CAD build for the part. Positions are in the model's coordinates, mm. A direction names the side the tool comes from. Give positions to 0.01 mm unless a question says otherwise; leave off trailing zeros. Loops run counter-clockwise (first coordinate to the right, second up) from the corner with the lowest first, then second, coordinate; pieces in that order, holes last.
Solid Edge part; units mm, degrees
sketch "Sketch1" plane through (0, 0, 0) normal (0, 0, 1) x (1, 0, 0)
  line L0 (-1.8475, 3.2) -> (1.8475, 3.2)
  line L1 (1.8475, 3.2) -> (3.695, 0)
  line L2 (3.695, 0) -> (1.8475, -3.2)
  line L3 (1.8475, -3.2) -> (-1.8475, -3.2)
  line L4 (-1.8475, -3.2) -> (-3.695, 0)
  line L5 (-3.695, 0) -> (-1.8475, 3.2)
extrude "Protrusion1" add sketch "Sketch1" along normal blind 0.5
sketch "Sketch2" plane through (0, 0, 0.5) normal (0, 0, 1) x (1, 0, 0)
  circle A0 centre (0, 0) radius 2.7
extrude "Ausprägung_2" add sketch "Sketch2" along normal blind 5.5
hole "Bohrung_1" at (0, 0, 6) direction (0, 0, -1) diameter 3 depth 5
chamfer "Fase_1" distance 0.5 angle 45 1 edges at (0, 1.5, 6)
1. Tool access for faces 5 (the face through (-0.585, 2.636, 3.212)), 6 (the face through (0, 0, 0)): list every direction of +Z, -Z, +X, -X, +Y, -Y with a clear straight run to the whole face (end or side of a thin tool).
Responses:
face 5: +Z
face 6: -Z, +X, -X, +Y, -Y
2. Drop flat-ended pins along their axis: pin 1 (2 mm diameter, centred on y = -0.5, z = 3.5, fed in from -X); pin 2 (2.5 mm diameter, centred on x = -0.5, y = 0.5, fed in from +Z). Give the stop position or say it passes through.
Responses:
pin 1: stops at x = -2.7
pin 2: stops at z = 5.96
3. Pull direction X, two halves, no side cores. Call faces 1 (the face through (-3, 0, 0.5)), 2 (the face through (2.784, -1.578, 0.246)), 3 (the face through (-0.07, 1.5, 3.22)), 4 (the face through (-2.784, 1.578, 0.246)): released by +X, released by -X, zero draft, split by the parting line, or undercut.
Responses:
face 1: zero draft
face 2: released by +X
face 3: undercut
face 4: released by -X
4. Saw through at B-B, the plane z = 2.25. List the corners of the cut face in (x, y), and give its area (3 significant figures).
Responses:
outline: circle Ø5.4 at (0, 0); hole circle Ø3 at (0, 0)
area: 15.8 mm2
5. Saw through at A-A, the plane x = 0. List the corners of the cut face in (y, z).
Responses:
outline: (-3.2, 0) - (3.2, 0) - (3.2, 0.5) - (2.7, 0.5) - (2.7, 6) - (2, 6) - (1.5, 5.5) - (1.5, 1) - (-1.5, 1) - (-1.5, 5.5) - (-2, 6) - (-2.7, 6) - (-2.7, 0.5) - (-3.2, 0.5) - close
6. Probe line 1 along Y through (x, z) = (0, 4.15); line 2 along Z through (x, y) = (2.25, -2); line 3 along X through (y, z) = (-1, 5.7). List the from-to ranges inside material, lowest first.
Responses:
line 1: y = -2.7 to -1.5, 1.5 to 2.7
line 2: z = 0 to 0.5
line 3: x = -2.51 to -1.37, 1.37 to 2.51
7. Saw through at C-C, the plane x = 3. List the corners of the cut face in (y, z), and give its area (3 significant figures).
Responses:
outline: (-1.2, 0) - (1.2, 0) - (1.2, 0.5) - (-1.2, 0.5) - close
area: 1.20 mm2
